from build123d import *

# Parameters (mm, degrees)
ESQUISSE2_R             = 3
BOSS_EXTRU_1_DEPTH      = 4
ESQUISSE3_R             = 1.5
ENL_V_MAT_EXTRU_1_DEPTH = 5
CONG_1_R                = 6.5
ESQUISSE4_W             = 4
ESQUISSE4_H             = 12
BOSS_EXTRU_2_DEPTH      = 4
CONG_2_R                = 5
ESQUISSE5_W             = 12
ESQUISSE5_H             = 4
ENL_V_MAT_EXTRU_2_DEPTH = 4
BOSS_EXTRU_3_START      = -2
BOSS_EXTRU_3_DEPTH      = 2
CONG_3_R                = 5
BOSS_EXTRU_4_DEPTH      = 2


with BuildPart() as part:
    # Esquisse2 → Boss.-Extru.1 (new body)
    with BuildSketch(Plane.XY):
        with BuildLine():
            Line((-199.971644797, -262.478940861), (-196.098548459, -348.633560192))
            ThreePointArc((-196.098548459, -348.633560192), (-8.923258694, -399.900456932), (180.352503917, -357.033575915))
            Line((180.352503917, -357.033575915), (187.115722814, -370.422335012))
            ThreePointArc((187.115722814, -370.422335012), (-9.257880895, -414.896724067), (-203.452244027, -361.707318699))
            Line((-203.452244027, -361.707318699), (-211.920441681, -376.762493353))
            ThreePointArc((-211.920441681, -376.762493353), (-226.337772202, -383.722686379), (-237.858405423, -372.606089933))
            ThreePointArc((-237.858405423, -372.606089933), (-265.801404699, -326.067035455), (-317.01741072, -308.077718418))
            ThreePointArc((-317.01741072, -308.077718418), (-326.924525304, -304.085923492), (-331.133147983, -294.268956483))
            Line((-331.133147983, -294.268956483), (-331.541895531, -264.271741188))
            Line((-331.541895531, -264.271741188), (-199.971644797, -262.478940861))
        make_face()
        with Locations((-317.134447512, -294.078207627)):
            Circle(ESQUISSE2_R, mode=Mode.SUBTRACT)
        with Locations((-212.300150205, -299.974825982)):
            Circle(ESQUISSE2_R, mode=Mode.SUBTRACT)
        with Locations((-224.122616287, -369.899044157)):
            Circle(ESQUISSE2_R, mode=Mode.SUBTRACT)
    extrude(amount=BOSS_EXTRU_1_DEPTH)

    # Esquisse3 → Enlèv. mat.-Extru.1 (cut, through all)
    with BuildSketch(Plane.XY.offset(4)):
        with BuildLine():
            ThreePointArc((180.352503917, -357.033575915), (175.075442806, -359.650649), (169.760416098, -362.18973084))
            ThreePointArc((169.760416098, -362.18973084), (179.734481353, -365.797780492), (176.126431702, -375.771845747))
            ThreePointArc((176.126431702, -375.771845747), (181.640771911, -373.137548338), (187.115722814, -370.422335012))
            Line((187.115722814, -370.422335012), (180.352503917, -357.033575915))
        make_face()
        with Locations((172.9434239, -368.980788294)):
            Circle(ESQUISSE3_R)
        with Locations((49.352874806, -404.5003631)):
            Circle(ESQUISSE3_R)
        with Locations((-79.152347286, -399.738859656)):
            Circle(ESQUISSE3_R)
        with Locations((-199.775396243, -355.170439446)):
            Circle(ESQUISSE3_R)
    extrude(amount=-ENL_V_MAT_EXTRU_1_DEPTH, mode=Mode.SUBTRACT)

    # Congé1
    cong_1_edges = [part.edges().sort_by_distance(p)[0] for p in [
        (-203.452244027, -361.707318699, 2),
        (-196.098548459, -348.633560192, 2),
    ]]
    fillet(cong_1_edges, radius=CONG_1_R)

    # Esquisse4 → Boss.-Extru.2 (add)
    with BuildSketch(Plane.XY.offset(4)):
        Polygon((-211.920441681, -376.762493353), (-223.686354588, -397.680506965), (-245.4759521, -385.424347686), (-237.96555462, -372.071996878), (-225.374330656, -376.762493353), align=None)
        Polygon((-238.339917634, -385.996197397), (-227.880910828, -391.879153851), (-225.919925343, -388.392818249), (-236.378932149, -382.509861795), align=None, mode=Mode.SUBTRACT)
        Polygon((-316.348629052, -308.074922938), (-340.348629052, -308.074922938), (-340.348629052, -283.074922938), (-331.285679934, -283.074922938), align=None)
        with Locations((-335.348629052, -295.574922938)):
            Rectangle(ESQUISSE4_W, ESQUISSE4_H, mode=Mode.SUBTRACT)
    extrude(amount=-BOSS_EXTRU_2_DEPTH)

    # Congé2
    cong_2_edges = [part.edges().sort_by_distance(p)[0] for p in [
        (-340.348629052, -308.074922938, 2),
        (-340.348629052, -283.074922938, 2),
        (-223.686354588, -397.680506965, 2),
        (-245.4759521, -385.424347686, 2),
        (-237.96555462, -372.071996878, 2),
    ]]
    fillet(cong_2_edges, radius=CONG_2_R)

    # Esquisse5 → Enlèv. mat.-Extru.2 (cut)
    with BuildSketch(Plane.XY.offset(4)):
        with Locations((-234.450045065, -274.867921079)):
            Rectangle(ESQUISSE5_W, ESQUISSE5_H)
    extrude(amount=-ENL_V_MAT_EXTRU_2_DEPTH, mode=Mode.SUBTRACT)

    # Esquisse6 → Boss.-Extru.3 (add)
    with BuildSketch(Plane.XY.offset(4).offset(BOSS_EXTRU_3_START)):
        with BuildLine():
            Line((169.003770429, -360.887760364), (169.760416098, -362.18973084))
            Line((169.760416098, -362.18973084), (178.042128837, -365.922078374))
            Line((178.042128837, -365.922078374), (179.374906332, -365.122545984))
            Line((179.374906332, -365.122545984), (173.538532023, -355.393623893))
            ThreePointArc((173.538532023, -355.393623893), (-12.898010177, -395.289629681), (-196.337202457, -343.324850443))
            Line((-196.337202457, -343.324850443), (-200.18270603, -348.6233841))
            Line((-200.18270603, -348.6233841), (-194.097457315, -353.368142853))
            Line((-194.097457315, -353.368142853), (-192.138010837, -349.120659359))
            ThreePointArc((-192.138010837, -349.120659359), (-12.977458778, -398.288633485), (169.003770429, -360.887760364))
        make_face()
    extrude(amount=-BOSS_EXTRU_3_DEPTH)

    # Congé3
    cong_3_edges = [part.edges().sort_by_distance(p)[0] for p in [
        (173.538532023, -355.393623893, 1),
    ]]
    fillet(cong_3_edges, radius=CONG_3_R)

    # Esquisse8 → Boss.-Extru.4 (add)
    with BuildSketch(Plane(origin=(0, 0, 0), x_dir=(-1, 0, 0), z_dir=(0, 0, -1))):
        Polygon((11.706214766, -405.333769301), (11.38055708, -395.339073354), (14.378965864, -395.241376048), (14.70462355, -405.236071995), align=None)
        Polygon((-83.101661868, -396.896225473), (-81.088533104, -387.100955565), (-78.149952132, -387.704894194), (-80.163080896, -397.500164102), align=None)
        Polygon((105.869114928, -391.438667615), (103.22261353, -381.795222673), (106.115647013, -381.001272254), (108.76214841, -390.644717196), align=None)
    extrude(amount=-BOSS_EXTRU_4_DEPTH)


solid = part.part
Could you check a few things on this model? Use its own coordinates, in mm. A direction names the side the tool comes from. Coordinates: 2 decimals unless noted, no trailing zeros. Order: outer loops, then holes, each group sorted by start corner. A loop starts at its lowest first (then second) coordinate and runs counter-clockwise, first axis right, second up.
Q1. Please list where these lines run through material, in increasing order: L1, parallel to Y at x = 94, z = 1.3; L2, parallel to Y at x = -117, z = 0.65; L3, parallel to Y at x = -202, z = 1.3.
Q2. Will these pins go through, and if not, where does the flat tip stop? pin 1 (8 mm diameter, centred on x = -5, y = -389.5, fed in from +Z); pin 2 (2 mm diameter, centred on x = -322, z = 2.5, fed in from -Y); pin 3 (1.2 mm diameter, centred on x = -234.5, z = 3, fed in from +Y); pin 4 (1.2 mm diameter, centred on x = -333, z = 1, fed in from +Y).
Q3. Thinking about a two-plate mould opening in X: for faces 1 (the cylindrical face through (125.58, -378.196, 1.014)), 2 (the flat face through (-178, -355, 0)), which applies, released by +X, released by -X, zero draft, split by the parting line, or undercut?
Q4. Suppose I cut it at B-B on x = -115.5. Please give me the cut outline in (y, z).
Q5. Suppose I cut it at C-C on z = 3.25. Give the number of separate pieces and of enclosed holes in the cut face, and give its area (3 significant figures).
Q6. Suppose I cut it at D-D on y = -334. Please give me the cut outline in (x, z).
Q7. Which directions (+Z, -Z, +X, -X, +Y, -Y) give clear straight access to the entire face, cutting with the end or side of a thin tool? Please do faces 3 (the cylindrical face through (-12.5, -395.302, 1.014)), 4 (the cylindrical face through (-151.13, -368.73, 1.01)), 5 (the flat face through (-9, -397, 2)).
Q8. Suppose I cut it at A-A on x = -176.5. Please give me the cut outline in (y, z), and give its area (3 significant figures).
Answer:
1. L1: y = -404.21 to -388.8, -387.25 to -384.17
1. L2: y = -398.17 to -382.51, -380.94 to -377.8
1. L3: y = -364.1 to -262.51
2. pin 1: passes through
2. pin 2: stops at y = -308.07
2. pin 3: stops at y = -262.94
2. pin 4: stops at y = -283.07
3. face 1: undercut
3. face 2: zero draft
4. outline: (-398.6, 0) - (-382.96, 0) - (-382.96, 4) - (-398.6, 4) - close; (-381.39, 0) - (-378.26, 0) - (-378.26, 2) - (-381.39, 2) - close
5. separate pieces: 1
5. enclosed holes: 10
5. area: 16,100 mm2
6. outline: (-257.39, 0) - (-196.76, 0) - (-196.76, 4) - (-257.39, 4) - close
7. face 3: +Z, -Z, +Y
7. face 4: +Z, -Z
7. face 5: +Z, +Y
8. outline: (-375.6, 0) - (-358.95, 0) - (-358.95, 4) - (-375.6, 4) - close; (-357.28, 0) - (-353.93, 0) - (-353.93, 2) - (-357.28, 2) - close
8. area: 73.3 mm2
